Drawing for the job (mm, zero at the part's lowest x, y, z). A direction names the side the tool comes from. Coordinates: 2 decimals unless noted, no trailing zeros. Write each loop counter-clockwise with the first axis right and the second up, starting at its lowest first coordinate (ties: lowest second). Pieces come first, ordered by that corner, then holes. Notation, with made-up numbers: M 30,81 L 85,81 A13 cw 85,106 Z; hole C 88.5,57.5 d10. An arc over 180 degrees is marked long. Use a Markdown table: item, result. Add a question column.
Q1. Tool access for the marked faces 1, 2, 3, 4 and 5: list every direction of +Z, -Z, +X, -X, +Y, -Y with a clear straight run to the whole face (end or side of a thin tool).
Q2. Pin check, flat tips, straight feed: pin 1 Ø1.5 at (y, z) = (59, 8.5) entering from +X; pin 2 Ø1.1 at (x, y) = (48.5, 63) entering from +Z; pin 3 Ø1 at (x, z) = (47.5, 4) entering from +Y; pin 4 Ø5 at (x, z) = (84.5, 8) entering from -Y (1 decimal). Stop position of each tip, or through.
Q3. Slice it at D-D on x = 8. Write the cut outline in (y, z), then the cut area to 3 significant figures.
Q4. Mould opens along Y. For the marked faces 6, 7, 8 and 9 say: released by +Y, released by -Y, zero draft, split by the parting line, or undercut.
Q5. Slice it at A-A on x = 62.5. Write the cut outline in (y, z), then the cut area to 3 significant figures.
Q6. Wall check: L1, parallel to Y at x = 75.5, z = 8; L2, parallel to Z at x = 8, y = 59.7; L3, parallel to Y at x = 63.5, z = 17.5. Give the ranges that are in metal, low to high. Write a range as from..to.
Q7. Slice it at C-C on z = 14.25. Write the cut outline in (x, y) (1 decimal), then the cut area to 3 significant figures.
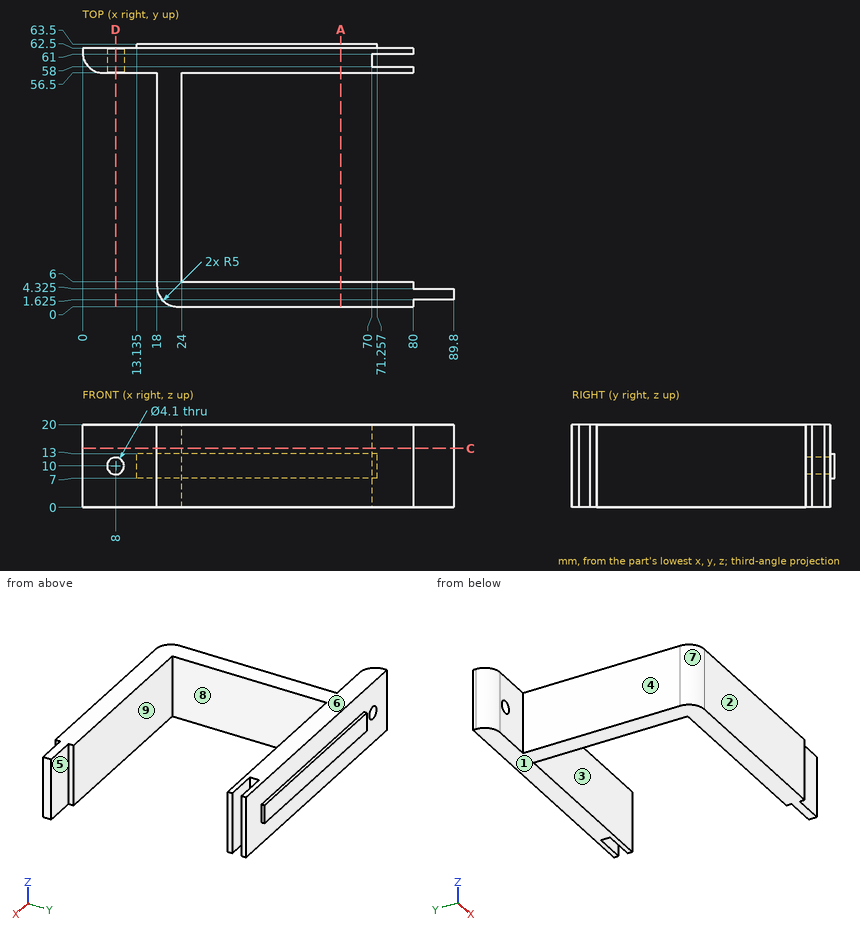
Recorded:
| question | item | result |
|---|---|---|
| 1 | face 1 | -Z, +X, -X, +Y, -Y |
| 1 | face 2 | +Z, -Z, +X, -X, -Y |
| 1 | face 3 | +Z, -Z, +X |
| 1 | face 4 | +Z, -Z, -X, -Y |
| 1 | face 5 | +Z, -Z, +X, +Y |
| 2 | pin 1 | x = 70 |
| 2 | pin 2 | z = 20 |
| 2 | pin 3 | y = 62.5 |
| 2 | pin 4 | y = 1.6 |
| 3 | outline | M 56.5,0 L 62.5,0 L 62.5,7.95 L 56.5,7.95 Z; M 56.5,12.05 L 62.5,12.05 L 62.5,20 L 56.5,20 Z |
| 3 | area | 95.4 mm² |
| 4 | face 6 | zero draft |
| 4 | face 7 | released by -Y |
| 4 | face 8 | undercut |
| 4 | face 9 | undercut |
| 5 | outline | M 0,0 L 6,0 L 6,20 L 0,20 Z; M 56.5,0 L 62.5,0 L 62.5,7 L 63.5,7 L 63.5,13 L 62.5,13 L 62.5,20 L 56.5,20 Z |
| 5 | area | 246 mm² |
| 6 | L1 | 0..6, 56.5..58, 61..62.5 |
| 6 | L2 | 0..7.95, 12.05..20 |
| 6 | L3 | 0..6, 56.5..62.5 |
| 7 | outline | M 0,61.5 A5 ccw 5,56.5 L 18,56.5 L 18,5 A5 ccw 23,0 L 80,0 L 80,1.6 L 89.8,1.6 L 89.8,4.3 L 80,4.3 L 80,6 L 24,6 L 24,56.5 L 80,56.5 L 80,58 L 70,58 L 70,61 L 80,61 L 80,62.5 L 0,62.5 Z |
| 7 | area | 1,140 mm² |
